```python
from build123d import *

# Parameters (mm, degrees)
SKETCH_R   = 15
SKETCH_R_2 = 6.25
PAD_DEPTH  = 8


with BuildPart() as part:
    # Sketch → Pad (new body)
    with BuildSketch(Plane.XY):
        with BuildLine():
            ThreePointArc((-7.543226, 16.892298), (-18.284536, -2.815273), (-2.1125, -18.378992))
            Line((-2.1125, -18.378992), (416.083897, -66.446904))
            ThreePointArc((416.083897, -66.446904), (420.501843, -66.131931), (424.504598, -64.235772))
            Line((424.504598, -64.235772), (471.738829, -29.940329))
            ThreePointArc((471.738829, -29.940329), (486.930116, -2.272998), (475.246411, 27.048452))
            Line((375.764429, 119.902673), (475.246411, 27.048452))
            ThreePointArc((375.764429, 119.902673), (364.508586, 127.107163), (351.427544, 129.84304))
            Line((259.292507, 132.108567), (351.427544, 129.84304))
            ThreePointArc((259.292507, 132.108567), (251.115722, 131.399038), (243.29653, 128.904344))
            Line((243.29653, 128.904344), (-7.543226, 16.892298))
        make_face()
        with Locations((304.622573, 100.984869)):
            Circle(SKETCH_R, mode=Mode.SUBTRACT)
        with Locations((365.151914, 52.530042)):
            Circle(SKETCH_R, mode=Mode.SUBTRACT)
        with Locations((333.42245, 78.605843)):
            Circle(SKETCH_R, mode=Mode.SUBTRACT)
        with Locations((417.454167, -54.525395)):
            Circle(SKETCH_R_2, mode=Mode.SUBTRACT)
        with Locations((130, -10)):
            Circle(SKETCH_R_2, mode=Mode.SUBTRACT)
        with Locations((155, 63)):
            Circle(SKETCH_R_2, mode=Mode.SUBTRACT)
        with Locations((39.52267, 6.161052)):
            Circle(SKETCH_R_2, mode=Mode.SUBTRACT)
        with Locations((402, 79)):
            Circle(SKETCH_R_2, mode=Mode.SUBTRACT)
        with BuildLine():
            ThreePointArc((5.221871, 0.542737), (-0.542737, 5.221871), (-5.221871, -0.542737))
            ThreePointArc((-5.221871, -0.542737), (0.542737, -5.221871), (5.221871, 0.542737))
        make_face(mode=Mode.SUBTRACT)
        with BuildLine():
            ThreePointArc((463.771661, -5.94486), (455.94486, 13.771661), (436.228339, 5.94486))
            ThreePointArc((436.228339, 5.94486), (444.05514, -13.771661), (463.771661, -5.94486))
        make_face(mode=Mode.SUBTRACT)
        with BuildLine():
            ThreePointArc((415.02967, 16.290529), (405.781984, 35.381896), (386.690617, 26.13421))
            ThreePointArc((386.690617, 26.13421), (395.938303, 7.042843), (415.02967, 16.290529))
        make_face(mode=Mode.SUBTRACT)
    extrude(amount=PAD_DEPTH)


solid = part.part
```
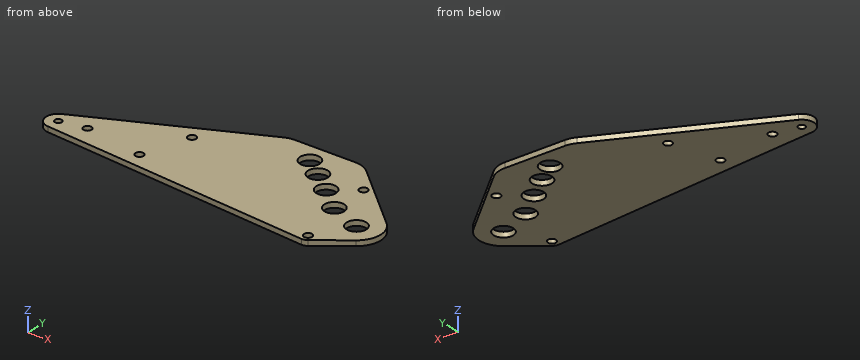
Input: part model. Units: mm. Frame: model coordinates. Give positions to 0.01 mm unless a question says otherwise; leave off trailing zeros. Order: outer loops, then holes, each group sorted by start corner. A loop starts at its lowest first (then second) coordinate and runs counter-clockwise, first axis right, second up. Notation, with made-up numbers: M 46.25,36 L 89.25,36 A30 cw 89.25,68 Z; hole C 53.5,-23 d2. An arc over 180 degrees is marked long. One line per question, with ' | ' between items. Start each with the question number.
1. Section query B-B (y = -10). Return the cut outline in (x, z), and give its area (3 significant figures).
2. Section query C-C (z = 2.25). Count the separate pieces of the cut face and the enclosed holes in it, and give its area (3 significant figures).
3. First-contact query: pin 1 Ø1.5 at (x, z) = (357.5, 2.5) entering from +Y. Flat tip, straight axial feed; report the tip coordinate or a pass-through.
4. Section query D-D (x = 402). Return the cut outline in (y, z).
5. Section query A-A (x = 130). Return the cut outline in (y, z), and give its area (3 significant figures).
6. Material intervals for probe 1 along X at (y, z) = (-0.5, 6.5); probe 2 along X at (y, z) = (73.5, 7); probe 3 along Y at (x, z) = (421.5, 3.5), sorted ascending. Write a range as [from, to].
Here are the results:
1) outline: M -15.56,0 L 123.75,0 L 123.75,8 L -15.56,8 Z; M 136.25,0 L 438.82,0 L 438.82,8 L 136.25,8 Z; M 461.18,0 L 485.62,0 L 485.62,8 L 461.18,8 Z | area: 3,730 mm²
2) separate pieces: 1 | enclosed holes: 11 | area: 60,000 mm²
3) pin 1: y = 129.33
4) outline: M -64.83,0 L 6.26,0 L 6.26,8 L -64.83,8 Z; M 36.17,0 L 72.75,0 L 72.75,8 L 36.17,8 Z; M 85.25,0 L 95.41,0 L 95.41,8 L 85.25,8 Z
5) outline: M -33.56,0 L -16.25,0 L -16.25,8 L -33.56,8 Z; M -3.75,0 L 78.31,0 L 78.31,8 L -3.75,8 Z | area: 795 mm²
6) probe 1: [-18.49, -5.23], [5.23, 435.01], [464.99, 487] | probe 2: [119.22, 319.32], [347.53, 399.03], [404.97, 425.48] | probe 3: [-65.82, -59.29], [-49.76, 77.21]
